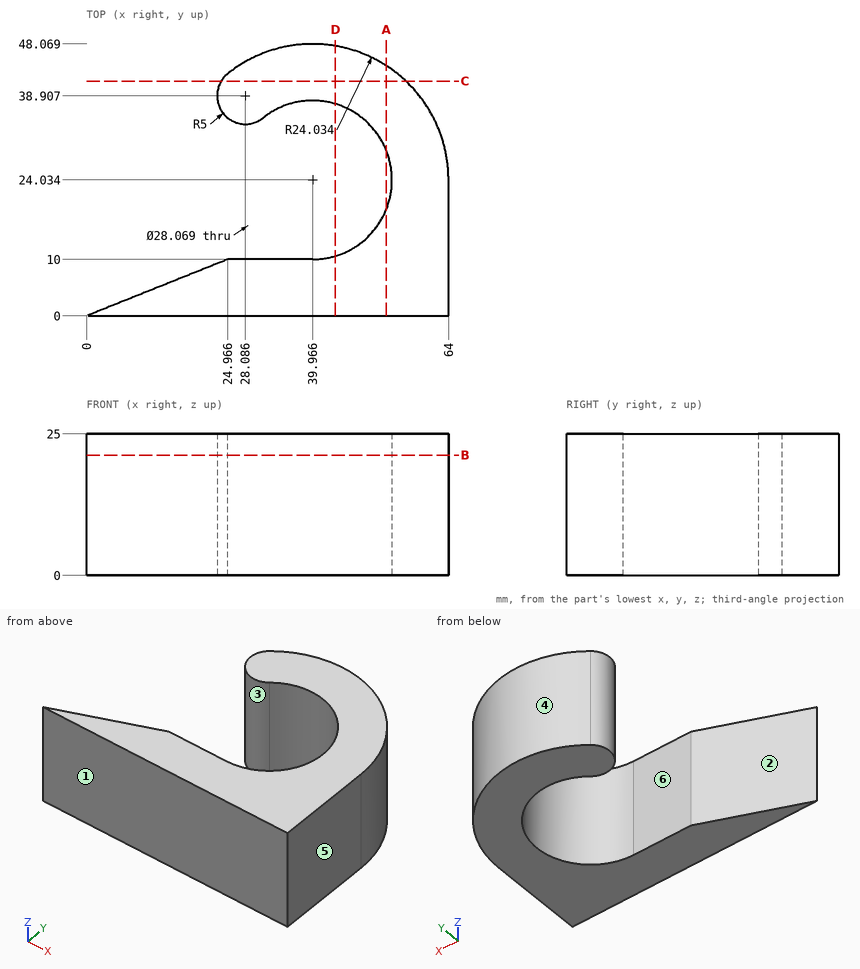
The drawing under review shows one solid part. Ordinate dimensions are in mm from its lowest x, y, z. A direction names the side the tool comes from. Give positions to 0.01 mm unless a question says otherwise; leave off trailing zeros. Loops run counter-clockwise (first coordinate to the right, second up) from the corner with the lowest first, then second, coordinate; pieces in that order, holes last. Notation, with made-up numbers: M 21.25,-12.75 L 63.25,-12.75 A7 ccw 63.25,-7.75 Z; hole C 78,17 d8. An arc over 180 degrees is marked long. One line per item, written item: value. Start each with the question number.
Q1. Add section D-D (x = 44). Give the boundary of the cut face in (y, z).
Q2. For L1, parallel to X at y = 35.5, z = 8.5 (1 decimal); L2, parallel to Y at x = 43, z = 21; L3, parallel to Y at x = 25.5, z = 1.5, list the stretches that pass through material, from the lowest coordinate up.
Q3. Machinability: for the marked faces 5 and 6, which of the approach directions +Z, -Z, +X, -X, +Y, -Y give a long, thin tool a straight path to every point of the face, cutting with its end or side? Answer none if there is none.
Q4. Add section B-B (z = 21.25). Give the boundary of the cut face in (x, y) (1 decimal), and give its area (3 significant figures).
Q5. Draft analysis for pull direction X (two halves, no side actions). For the marked faces 1, 2, 3 and 4, state which applies: released by +X, released by -X, zero draft, split by the parting line, or undercut.
Q6. Clearance check with flat-ended pins moving along their axes: pin 1 Ø12 at (x, y) = (38, 18.5) entering from -Z; pin 2 Ø1.5 at (x, z) = (12, 18.5) entering from +Y; pin 3 Ø5 at (y, z) = (10.5, 15) entering from -X (1 decimal); pin 4 Ø12 at (x, z) = (29, 16.5) entering from +Y. State where each tip first meets the part, or that it passes through.
Q7. Add section C-C (y = 41.5). Give the boundary of the cut face in (x, z), and give its area (3 significant figures).
Q8. Add section A-A (x = 53). Give the boundary of the cut face in (y, z).
Reply:
1. outline: M 0,0 L 10.59,0 L 10.59,25 L 0,25 Z; M 37.48,0 L 47.73,0 L 47.73,25 L 37.48,25 Z
2. L1: 24.4 to 31.9, 48.1 to 61.1
2. L2: 0 to 10.33, 37.74 to 47.88
2. L3: 0 to 10, 34.63 to 43.23
3. face 5: +Z, -Z, +X, +Y, -Y
3. face 6: +Z, -Z, -X
4. outline: M 0,0 L 64,0 L 64,24 A24 ccw 25,42.8 A5 ccw 31.2,35 A14 cw long 40,10 L 25,10 Z
4. area: 1,160 mm²
5. face 1: zero draft
5. face 2: released by -X
5. face 3: undercut
5. face 4: split by the parting line
6. pin 1: through
6. pin 2: y = 5.11
6. pin 3: x = 20
6. pin 4: y = 47.55
7. outline: M 23.81,0 L 56.48,0 L 56.48,25 L 23.81,25 Z
7. area: 817 mm²
8. outline: M 0,0 L 18.83,0 L 18.83,25 L 0,25 Z; M 29.24,0 L 44.23,0 L 44.23,25 L 29.24,25 Z
